For this review, take the finished solid that the model builds, in its own axes (mm). A direction names the side the tool comes from. Coordinates: 2 decimals unless noted, no trailing zeros. Loops run counter-clockwise (first coordinate to the right, second up) from the corner with the lowest first, then second, coordinate; pieces in that order, holes last.
1. Machinability: for faces 4 (the face through (-16, -1.588, 4)), 5 (the face through (-19.74, -12.678, 5.114)), which of the approach directions +Z, -Z, +X, -X, +Y, -Y give a long, thin tool a straight path to every point of the face, cutting with its end or side? Answer none if there is none.
2. Take a section at A-A, the plane z = 0. Count the separate pieces of the cut face and the enclosed holes in it, then the cut area to 3 significant figures.
3. To check wall thickness, follow probe 1 along X at (y, z) = (-6.5, 0); probe 2 along Y at (x, z) = (19.5, 2.5); probe 3 along X at (y, z) = (-9.5, -10). State the ranges of each line that lie inside material, in increasing order.
4. Clearance check with flat-ended pins moving along their axes: P1, Ø9, axis at x = 23.5, z = 0, coming from the +Y side; P2, Ø4, axis at x = 21, z = 6, coming from the +Y side; P3, Ø5, axis at y = -11, z = -11.5, coming from the -X side. State where each tip first meets the part, or that it passes through.
5. Take a section at D-D, the plane y = -4.5. State the section outline as (x, z) points.
6. Take a section at C-C, the plane x = 0. State the section outline as (y, z) points.
7. Mouldability with a two-part tool opening along Z and no side actions: class faces 1 (the face through (19.74, -12.678, -5.114)), 2 (the face through (-15.87, -0.78, -3.52)), 3 (the face through (27.304, -12.678, 0.091)) as pulls with the +Z half, pulls with the -Z half, needs draft (parallel to the pull), parting line crosses it, or undercut.
```python
from build123d import *
from build123d.topology import SkipClean

# Parameters (mm, degrees)
SKETCH1_R             = 19.05
SKETCH1_R_2           = 16.256
BOSS_EXTRUDE1_DEPTH   = 1.5875
SKETCH2_R             = 19.05
SKETCH2_R_2           = 16.66875
BOSS_EXTRUDE2_DEPTH   = 9.525
CHAMFER1_SIZE         = 1.27
SKETCH3_R             = 16.66875
BOSS_EXTRUDE3_DEPTH   = 3.175
FILLET1_R             = 6.35
F_6_CLEARANCE_HOLE1_D = 4.3053


with BuildPart() as part:
    # Sketch1 → Boss-Extrude1 (new body)
    with BuildSketch(Plane(origin=(0, 0, 0), x_dir=(1, 0, 0), z_dir=(0, 1, 0))):
        with Locations(Location((0, 0, 0), (0, 0, 270))):
            Circle(SKETCH1_R)
        with Locations(Location((0, 0, 0), (0, 0, 270))):
            Circle(SKETCH1_R_2, mode=Mode.SUBTRACT)
    extrude(amount=-BOSS_EXTRUDE1_DEPTH)

    # Sketch2 → Boss-Extrude2 (add)
    with BuildSketch(Plane.XZ.offset(1.5875)):
        with Locations(Location((0, 0, 0), (0, 0, 90))):
            Circle(SKETCH2_R)
        with Locations(Location((0, 0, 0), (0, 0, 270))):
            Circle(SKETCH2_R_2, mode=Mode.SUBTRACT)
    extrude(amount=BOSS_EXTRUDE2_DEPTH)

    # Chamfer1
    chamfer1_edges = [part.edges().sort_by_distance(p)[0] for p in [
        (0, 0, -19.05),
    ]]
    chamfer(chamfer1_edges, length=CHAMFER1_SIZE)

    # Sketch3 → Boss-Extrude3 (add)
    with SkipClean():  # the faces are left unmerged after this step: merging them gives an invalid solid
        with BuildSketch(Plane.XZ.offset(11.1125)):
            with BuildLine():
                Line((-23.1775, 4.1275), (-18.5974795, 4.1275))
                ThreePointArc((-18.5974795, 4.1275), (0, 19.05), (18.5974795, 4.1275))
                Line((18.5974795, 4.1275), (23.1775, 4.1275))
                ThreePointArc((23.1775, 4.1275), (27.305, 0), (23.1775, -4.1275))
                Line((23.1775, -4.1275), (18.5974795, -4.1275))
                ThreePointArc((18.5974795, -4.1275), (0, -19.05), (-18.5974795, -4.1275))
                Line((-18.5974795, -4.1275), (-23.1775, -4.1275))
                ThreePointArc((-23.1775, -4.1275), (-27.305, 0), (-23.1775, 4.1275))
            make_face()
            with Locations(Location((0, 0, 0), (0, 0, 270))):
                Circle(SKETCH3_R, mode=Mode.SUBTRACT)
        extrude(amount=BOSS_EXTRUDE3_DEPTH)
    add(part.part.scale(1), mode=Mode.REPLACE)  # the faces are merged on a copy

    # Fillet1
    # the kernel refuses this fillet: 6.35 mm, written as the material it adds along each edge
    with BuildSketch(Plane(origin=(18.5974795, -11.1125, 4.1275), x_dir=(-0.3162725181456123, 0, 0.948668379501411), z_dir=(0, -1, 0)), Plane(origin=(-18.5974795, -11.1125, -4.1275), x_dir=(0.3162725181456131, 0, -0.9486683795014108), z_dir=(0, -1, 0))) as fillet1_piece_1:
        with BuildLine():
            CenterArc((4.587900184, -6.316085186), FILLET1_R, 95.924326289, 65.63802206)
            Line((-1.436144025, -4.307754696), (0, 0))
            ThreePointArc((0, 0), (1.966242936, -0.101744441), (3.932485872, 0))
        make_face()
    extrude(amount=3.175)
    with BuildSketch(Plane(origin=(-18.5974795, -11.1125, 4.1275), x_dir=(0.3162725181456136, 0, 0.9486683795014107), z_dir=(0, -1, 0)), Plane(origin=(18.5974795, -11.1125, -4.1275), x_dir=(-0.3162725181456148, 0, -0.9486683795014103), z_dir=(0, -1, 0))) as fillet1_piece_2:
        with BuildLine():
            CenterArc((4.587900184, 6.316085186), FILLET1_R, 198.437651651, 65.63802206)
            Line((-1.436144025, 4.307754696), (0, 0))
            ThreePointArc((0, 0), (1.966242936, 0.101744441), (3.932485872, 0))
        make_face()
    extrude(amount=3.175)

    # #6 Clearance Hole1 (through all)
    with Locations(Plane(origin=(0, -14.2875, 0), x_dir=(-1, 0, 0), z_dir=(0, -1, 0))):
        with Locations((-23.1775, 0), (23.1775, 0)):
            Hole(F_6_CLEARANCE_HOLE1_D / 2)


solid = part.part
```
Results list:
1. face 4: -Y
1. face 5: +Z, -X, +Y, -Y
2. separate pieces: 4
2. enclosed holes: 0
2. area: 92.8 mm2
3. probe 1: x = -19.05 to -16.67, 16.67 to 19.05
3. probe 2: y = -14.29 to -11.11
3. probe 3: x = -16.21 to -13.34, 13.34 to 16.21
4. P1: stops at y = -1.22
4. P2: stops at y = -11.11
4. P3: stops at x = -16.79
5. outline: circle Ø38.1 at (0, 0); hole circle Ø33.34 at (0, 0)
6. outline: (-14.29, -19.05) - (-1.27, -19.05) - (0, -17.78) - (0, -16.26) - (-1.59, -16.26) - (-1.59, -16.67) - (-14.29, -16.67) - close; (-14.29, 16.67) - (-1.59, 16.67) - (-1.59, 16.26) - (0, 16.26) - (0, 17.78) - (-1.27, 19.05) - (-14.29, 19.05) - close
7. face 1: pulls with the -Z half
7. face 2: undercut
7. face 3: parting line crosses it
